from build123d import *

# Parameters (mm, degrees)
CROQUIS1_R              = 1.7
SALIENTE_EXTRUIR1_DEPTH = 3
CORTAR_EXTRUIR1_REACH   = 88.406
CROQUIS3_W              = 4
CROQUIS3_H              = 2
CROQUIS3_W_2            = 10
CROQUIS3_H_2            = 5.9


with BuildPart() as part:
    # Croquis1 → Saliente-Extruir1 (new body)
    with BuildSketch(Plane(origin=(0, 0, 0), x_dir=(1, 0, 0), z_dir=(0, 1, 0))):
        with BuildLine():
            Line((-29.607107898, -53.127168991), (-29.822053636, -53.49946593))
            ThreePointArc((-29.822053636, -53.49946593), (-31.312291696, -54.787421208), (-33.280086565, -54.873570042))
            ThreePointArc((-33.280086565, -54.873570042), (-40.509483904, -58.24573384), (-38, -65.817930688))
            ThreePointArc((-38, -65.817930688), (0, -76), (38, -65.817930688))
            ThreePointArc((38, -65.817930688), (40.509483904, -58.24573384), (33.280086565, -54.873570042))
            ThreePointArc((33.280086565, -54.873570042), (31.312291696, -54.787421208), (29.822053636, -53.49946593))
            Line((29.822053636, -53.49946593), (29.607107898, -53.127168991))
            ThreePointArc((29.607107898, -53.127168991), (27.954273423, -51.77997422), (25.823903289, -51.871180841))
            ThreePointArc((25.823903289, -51.871180841), (0, -57.458865486), (-25.823903289, -51.871180841))
            ThreePointArc((-25.823903289, -51.871180841), (-27.954273423, -51.77997422), (-29.607107898, -53.127168991))
        make_face()
        with Locations(Location((27.009031687, -54.627168991, 0), (0, 0, 270))):
            Circle(CROQUIS1_R, mode=Mode.SUBTRACT)
        with Locations(Location((0, -61.515130262, 0), (0, 0, 270))):
            Circle(CROQUIS1_R, mode=Mode.SUBTRACT)
        with Locations(Location((-27.009031687, -54.627168991, 0), (0, 0, 270))):
            Circle(CROQUIS1_R, mode=Mode.SUBTRACT)
    extrude(amount=SALIENTE_EXTRUIR1_DEPTH)

    # Croquis3 → Cortar-Extruir1 (cut, up to next)
    with BuildSketch(Plane.XZ, mode=Mode.PRIVATE) as cortar_extruir1_sk1:
        with Locations((15, 70)):
            Rectangle(CROQUIS3_W, CROQUIS3_H)
    cortar_extruir1_tool1 = extrude(cortar_extruir1_sk1.sketch, amount=-CORTAR_EXTRUIR1_REACH, mode=Mode.PRIVATE) & part.part
    # Croquis3 → Cortar-Extruir1 (cut, up to next)
    with BuildSketch(Plane.XZ, mode=Mode.PRIVATE) as cortar_extruir1_sk2:
        with Locations((0, 70.05)):
            Rectangle(CROQUIS3_W_2, CROQUIS3_H_2)
    cortar_extruir1_tool2 = extrude(cortar_extruir1_sk2.sketch, amount=-CORTAR_EXTRUIR1_REACH, mode=Mode.PRIVATE) & part.part
    # Croquis3 → Cortar-Extruir1 (cut, up to next)
    with BuildSketch(Plane.XZ, mode=Mode.PRIVATE) as cortar_extruir1_sk3:
        with Locations((-15, 70)):
            Rectangle(CROQUIS3_W, CROQUIS3_H)
    cortar_extruir1_tool3 = extrude(cortar_extruir1_sk3.sketch, amount=-CORTAR_EXTRUIR1_REACH, mode=Mode.PRIVATE) & part.part
    add(cortar_extruir1_tool1.solids().sort_by_distance((15, 0, 70))[0], mode=Mode.SUBTRACT)
    add(cortar_extruir1_tool2.solids().sort_by_distance((0, 0, 70.05))[0], mode=Mode.SUBTRACT)
    add(cortar_extruir1_tool3.solids().sort_by_distance((-15, 0, 70))[0], mode=Mode.SUBTRACT)


solid = part.part
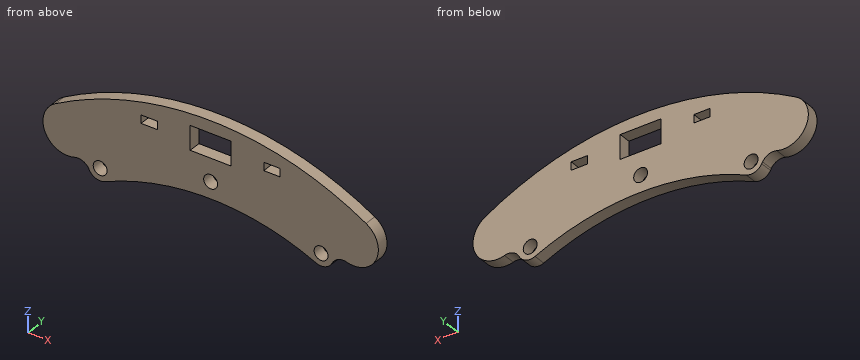
Here's how the part is built. I have some questions about the finished solid (model axes, mm). Give positions to 0.01 mm unless a question says otherwise; leave off trailing zeros. Loops run counter-clockwise (first coordinate to the right, second up) from the corner with the lowest first, then second, coordinate; pieces in that order, holes last. Notation, with made-up numbers: (-29, 48.5) -> (30, 48.5) arc R10 ccw to (30, 63.5) -> close; hole circle Ø8 at (46.25, 49.25). An arc over 180 degrees is marked (long way). Answer as a JSON object with one key per item and string values. Group by question number.
Item 1: Imagine slicing it at A-A on x = 0. Write out the boundary of the cut face in (y, z), then the cut area to 3 significant figures.
Item 2: Imagine slicing it at B-B on x = 15.5. Write out the boundary of the cut face in (y, z).
Item 3: I need wall thicknesses on L1, parallel to X at y = 1.55, z = 60.5; L2, parallel to X at y = 0.2, z = 68.5; L3, parallel to Z at x = -16.5, y = 1. Which ranges of each line are inside material? Lowest first, please.
Item 4: Imagine slicing it at C-C on y = 1.5. Write out the boundary of the cut face in (x, z), then the cut area to 3 significant figures.
Item 5: Will these pins go through, and if not, where does the flat tip stop? pin 1 (1.5 mm diameter, centred on y = 2, z = 69.5, fed in from +X) (3 decimals); pin 2 (1.5 mm diameter, centred on x = 14.5, y = 1.5, fed in from +Z); pin 3 (1.5 mm diameter, centred on x = -15.5, y = 1.5, fed in from -Z); pin 4 (3 mm diameter, centred on x = -27.01, z = 54.63, fed in from -Y).
Item 6: Imagine slicing it at D-D on x = -12. Write out the boundary of the cut face in (y, z), then the cut area to 3 significant figures.
Answer list:
{
 "1": {"outline": "(0, 57.46) -> (3, 57.46) -> (3, 59.82) -> (0, 59.82) -> close; (0, 63.22) -> (3, 63.22) -> (3, 67.1) -> (0, 67.1) -> close; (0, 73) -> (3, 73) -> (3, 76) -> (0, 76) -> close", "area": "27.7 mm2"},
 "2": {"outline": "(0, 55.51) -> (3, 55.51) -> (3, 69) -> (0, 69) -> close; (0, 71) -> (3, 71) -> (3, 74.4) -> (0, 74.4) -> close"},
 "3": {"L1": "x = -41 to -1.36, 1.36 to 41", "L2": "x = -32.92 to -5, 5 to 32.92", "L3": "z = 55.24 to 69, 71 to 74.19"},
 "4": {"outline": "(-38, 65.82) arc R6 ccw to (-33.28, 54.87) arc R3 cw to (-29.82, 53.5) -> (-29.61, 53.13) arc R3 ccw to (-25.82, 51.87) arc R62.47 cw to (25.82, 51.87) arc R3 ccw to (29.61, 53.13) -> (29.82, 53.5) arc R3 cw to (33.28, 54.87) arc R6 ccw to (38, 65.82) arc R76 ccw to start; hole circle Ø3.4 at (-27.01, 54.63); hole (-17, 69) -> (-13, 69) -> (-13, 71) -> (-17, 71) -> close; hole (-5, 67.1) -> (5, 67.1) -> (5, 73) -> (-5, 73) -> close; hole circle Ø3.4 at (0, 61.52); hole (13, 69) -> (17, 69) -> (17, 71) -> (13, 71) -> close; hole circle Ø3.4 at (27.01, 54.63)", "area": "1,280 mm2"},
 "5": {"pin 1": "stops at x = 32.395", "pin 2": "stops at z = 74.75", "pin 3": "stops at z = 55.31", "pin 4": "passes through"},
 "6": {"outline": "(0, 56.3) -> (3, 56.3) -> (3, 75.05) -> (0, 75.05) -> close", "area": "56.3 mm2"}
}
